Source: three-view drawing plus pictorial views. Frame: mm from the lowest corner of the part. Coordinates: 2 decimals unless noted, no trailing zeros. Order: outer loops, then holes, each group sorted by start corner. A loop starts at its lowest first (then second) coordinate and runs counter-clockwise, first axis right, second up. Notation, with made-up numbers: (-33, 66) -> (-3, 66) arc R13 cw to (-3, 89) -> close; hole circle Ø6 at (28.25, 76.5). An arc over 180 degrees is marked (long way). Use one line per item in the form item = value. Start each with the question number.
1) Section query B-B on y = 74.5. Output: boundary loops of the cut face in (x, z).
2) Ray query, line 1 along Y through (x, z) = (6, 2.5); line 2 along X through (y, z) = (139, 2.3); line 3 along Y through (x, z) = (118.2, 1.45). Return the intervals inside material, ascending.
3) Section query C-C on z = 2.85. Count the separate pieces of the cut face and the enclosed holes in it, then the cut area to 3 significant figures.
4) Section query A-A on x = 153. Output: boundary loops of the cut face in (y, z), then the cut area to 3 significant figures.
5) Pin query (flat end, axial travel): pin 1 (1.2 mm diameter, centred on x = 119, z = 2.5, fed in from -Y). Return the tip coordinate at first contact, or that it passes through.
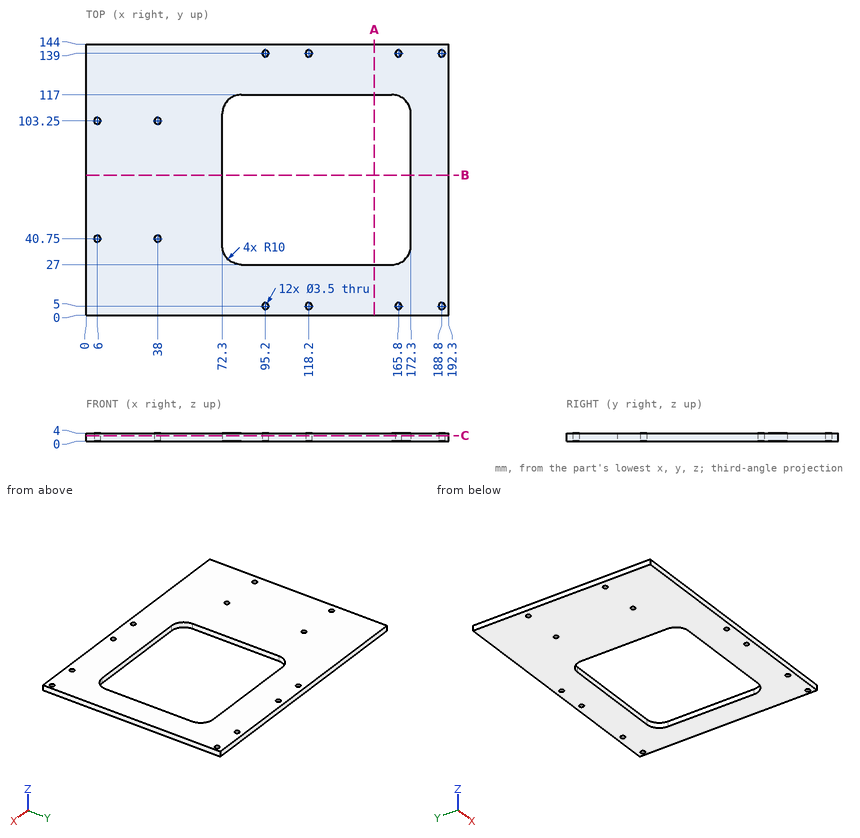
Answers below:
q1.outline = (0, 0) -> (72.3, 0) -> (72.3, 4) -> (0, 4) -> close; (172.3, 0) -> (192.3, 0) -> (192.3, 4) -> (172.3, 4) -> close
q2.line_1 = 0 to 39, 42.5 to 101.5, 105 to 144
q2.line_2 = 0 to 93.45, 96.95 to 116.45, 119.95 to 164.05, 167.55 to 187.05, 190.55 to 192.3
q2.line_3 = 0 to 3.25, 6.75 to 27, 117 to 137.25, 140.75 to 144
q3.separate_pieces = 1
q3.enclosed_holes = 13
q3.area = 18,700 mm^2
q4.outline = (0, 0) -> (27, 0) -> (27, 4) -> (0, 4) -> close; (117, 0) -> (144, 0) -> (144, 4) -> (117, 4) -> close
q4.area = 216 mm^2
q5.pin_1 = 0
